Read the model definition and answer for the solid it produces. Units are mm, in the model's axes. A direction names the side the tool comes from. Coordinates: 2 decimals unless noted, no trailing zeros. Order: outer loops, then holes, each group sorted by start corner. A loop starts at its lowest first (then second) coordinate and runs counter-clockwise, first axis right, second up. Notation, with made-up numbers: M 2.25,54 L 50.25,54 A32 ccw 50.25,88 Z; hole C 16,9.5 d11. An arc over 180 degrees is marked long. Use a Markdown table: item, result. Add a question column.
1) Find section C-C on x = -38.5. Write down the section's boundary in (y, z), plus the area to 3 significant figures.
2) For faces 4 (the face through (-61, 60.108, 26)), 5 (the face through (-21.845, 14, 5)), 6 (the face through (-2, 87.208, 1)), determine the directions among +Z, -Z, +X, -X, +Y, -Y from which every point of the face is accessible in a straight line to the end or side of a thin tool.
3) Find section D-D on y = -34.5. Write down the section's boundary in (x, z).
4) Find section A-A on z = 43.5. Write down the section's boundary in (x, y), plus the area to 3 significant figures.
5) Find section B-B on y = -15.5. Write down the section's boundary in (x, z).
6) The mould has two halves that part along X. Classify faces 1 (the face through (-3, 18, 3)), 2 (the face through (-62.218, 14.974, 24.65)), 3 (the face through (57.222, 14.882, 24.65)): released by +X, released by -X, zero draft, split by the parting line, or undercut.
7) Each of these flat-tipped pins is pushed along its axis until it touches: pin 1 Ø1.6 at (x, y) = (18, 1) entering from +Z; pin 2 Ø1.6 at (x, z) = (-23, 5) entering from +Y; pin 3 Ø2.5 at (x, z) = (56.5, 22) entering from +Y. Where does it stop, or does it pass through?
8) Find the intervals of material crossed by probe 1 along X at (y, z) = (23.5, 10); probe 2 along Z at (x, y) = (0.5, 57); probe 3 along Y at (x, z) = (12, 19), in increasing order. Write a range as [from, to].
from build123d import *

# Parameters (mm, degrees)
F0_W     = 2
F0_H     = 85
F0_W_2   = 3.0000019335
F0_H_2   = 27.1
F1_DEPTH = 3
F2_DEPTH = 50
F3_DEPTH = 8


# Not quite as in the source:
# - ends of sketch curves that miss each other by under 0.0002 mm in the source are joined


with BuildPart() as f1:
    # F0 (on Top) → F1 (new body)
    with BuildSketch(Plane.XY):
        with BuildLine():
            Line((54.5097446937, 40.5472581927), (54.5097446937, 60.1075036168))
            Line((54.5097446937, 60.1075036168), (54.5097446937, 87.2075036168))
            Line((54.5097446937, 87.2075036168), (-59.4902514393, 87.2075036168))
            Line((-59.4902514393, 87.2075036168), (-59.4902514393, 60.1075036168))
            Line((-59.4902514393, 60.1075036168), (-59.4902514393, 40.5472581927))
            Line((-59.4902514393, 40.5472581927), (-59.4902514393, 18.2598339378))
            ThreePointArc((-59.4902514393, 18.2598339378), (-59.2538728212, 15.4347680531), (-58.5513104793, 12.6882651386))
            Line((-58.5513104793, 12.6882651386), (-40.5146915017, -37.5214353961))
            ThreePointArc((-40.5146915017, -37.5214353961), (-30.4754938788, -48.962906346), (-15.8429778585, -53.1560222908))
            Line((-15.8429778585, -53.1560222908), (10.8692885058, -53.1560668961))
            ThreePointArc((10.8692885058, -53.1560668961), (25.4978663276, -48.9610815315), (35.534184756, -37.5214353961))
            Line((35.534184756, -37.5214353961), (53.5708037336, 12.6882651386))
            ThreePointArc((53.5708037336, 12.6882651386), (54.2733660755, 15.4347680531), (54.5097446937, 18.2598339378))
            Line((54.5097446937, 18.2598339378), (54.5097446937, 40.5472581927))
        make_face()
        with Locations((-22.8452533728, 14.6164752861)):
            Rectangle(F0_W, F0_H, mode=Mode.SUBTRACT)
        with Locations((17.8647466272, 14.6164752861)):
            Rectangle(F0_W, F0_H, mode=Mode.SUBTRACT)
        with Locations((-60.9902524061, 73.6575036168)):
            Rectangle(F0_W_2, F0_H_2)
        with Locations((56.0097456604, 73.6575036168)):
            Rectangle(F0_W_2, F0_H_2)
    extrude(amount=F1_DEPTH)

    # F0 (on Top) → F2 (join)
    with BuildSketch(Plane.XY):
        with BuildLine():
            Line((-15.8404213062, -56.156068814), (10.8599145605, -56.1560242285))
            ThreePointArc((10.8599145605, -56.1560242285), (27.1664180437, -51.4552481906), (38.3132826454, -38.6588744882))
            Line((38.3132826454, -38.6588744882), (56.3994961696, 11.6888855872))
            ThreePointArc((56.3994961696, 11.6888855872), (57.2302307851, 14.9277918348), (57.5097466272, 18.2598339378))
            Line((57.5097466272, 18.2598339378), (57.5097466272, 40.2075055503))
            Line((57.5097466272, 40.2075055503), (57.5097466272, 60.1075036168))
            Line((57.5097466272, 60.1075036168), (54.5097446937, 60.1075036168))
            Line((54.5097446937, 60.1075036168), (54.5097446937, 40.5472581927))
            Line((54.5097446937, 40.5472581927), (54.5097446937, 18.2598339378))
            ThreePointArc((54.5097446937, 18.2598339378), (54.2733660755, 15.4347680531), (53.5708037336, 12.6882651386))
            Line((53.5708037336, 12.6882651386), (35.534184756, -37.5214353961))
            ThreePointArc((35.534184756, -37.5214353961), (25.4978663276, -48.9610815315), (10.8692885058, -53.1560668961))
            Line((10.8692885058, -53.1560668961), (-15.8429778585, -53.1560222908))
            ThreePointArc((-15.8429778585, -53.1560222908), (-30.4754938788, -48.962906346), (-40.5146915017, -37.5214353961))
            Line((-40.5146915017, -37.5214353961), (-58.5513104793, 12.6882651386))
            ThreePointArc((-58.5513104793, 12.6882651386), (-59.2538728212, 15.4347680531), (-59.4902514393, 18.2598339378))
            Line((-59.4902514393, 18.2598339378), (-59.4902514393, 40.5472581927))
            Line((-59.4902514393, 40.5472581927), (-59.4902514393, 60.1075036168))
            Line((-59.4902514393, 60.1075036168), (-62.4902533728, 60.1075036168))
            Line((-62.4902533728, 60.1075036168), (-62.4902533728, 40.2075055503))
            Line((-62.4902533728, 40.2075055503), (-62.4902533728, 18.2598339378))
            ThreePointArc((-62.4902533728, 18.2598339378), (-62.2107375308, 14.9277918348), (-61.3800029152, 11.6888855872))
            Line((-61.3800029152, 11.6888855872), (-43.293789391, -38.6588744882))
            ThreePointArc((-43.293789391, -38.6588744882), (-32.1469247894, -51.4552481906), (-15.8404213062, -56.156068814))
        make_face()
    extrude(amount=F2_DEPTH)

    # F0 (on Top) → F3 (join)
    with BuildSketch(Plane.XY):
        with Locations((17.8647466272, 14.6164752861)):
            Rectangle(F0_W, F0_H)
        with Locations((-22.8452533728, 14.6164752861)):
            Rectangle(F0_W, F0_H)
    extrude(amount=F3_DEPTH)


solid = f1.part
Check result:
| question | item | result |
|---|---|---|
| 1 | outline | M -46.03,0 L 87.21,0 L 87.21,3 L -41.12,3 L -41.12,50 L -46.03,50 Z |
| 1 | area | 630 mm2 |
| 2 | face 4 | +Z, +X, -X, +Y |
| 2 | face 5 | +Z, +Y |
| 2 | face 6 | +Z, -Z, +X, -X, +Y |
| 3 | outline | M -44.79,0 L 39.81,0 L 39.81,50 L 36.62,50 L 36.62,3 L -41.6,3 L -41.6,50 L -44.79,50 Z |
| 4 | outline | M -62.49,18.26 A20 ccw -61.38,11.69 L -43.29,-38.66 A30 ccw -15.84,-56.16 L 10.86,-56.16 A30 ccw 38.31,-38.66 L 56.4,11.69 A20 ccw 57.51,18.26 L 57.51,60.11 L 54.51,60.11 L 54.51,18.26 A17 cw 53.57,12.69 L 35.53,-37.52 A27 cw 10.87,-53.16 L -15.84,-53.16 A27 cw -40.51,-37.52 L -58.55,12.69 A17 cw -59.49,18.26 L -59.49,60.11 L -62.49,60.11 Z |
| 4 | area | 885 mm2 |
| 5 | outline | M -51.61,0 L 46.63,0 L 46.63,50 L 43.44,50 L 43.44,3 L 18.86,3 L 18.86,8 L 16.86,8 L 16.86,3 L -21.85,3 L -21.85,8 L -23.85,8 L -23.85,3 L -48.43,3 L -48.43,50 L -51.61,50 Z |
| 6 | face 1 | undercut |
| 6 | face 2 | released by -X |
| 6 | face 3 | released by +X |
| 7 | pin 1 | stops at z = 8 |
| 7 | pin 2 | stops at y = 57.12 |
| 7 | pin 3 | stops at y = 60.11 |
| 8 | probe 1 | x = [-62.49, -59.49], [54.51, 57.51] |
| 8 | probe 2 | z = [0, 3] |
| 8 | probe 3 | y = [-56.14, -53.14] |
